Geometry check sheet. Reference: drawing and pictorial views, mm from the part's lowest x, y, z. Give positions to 0.01 mm unless a question says otherwise; leave off trailing zeros. Order: outer loops, then holes, each group sorted by start corner. A loop starts at its lowest first (then second) coordinate and runs counter-clockwise, first axis right, second up. Notation, with made-up numbers: M 85,-33.75 L 104,-33.75 A15 ccw 104,-8.75 Z; hole C -9,54 d2. An arc over 180 degrees is marked long. Answer as a JSON object with one key per item and string values. Group by question number.
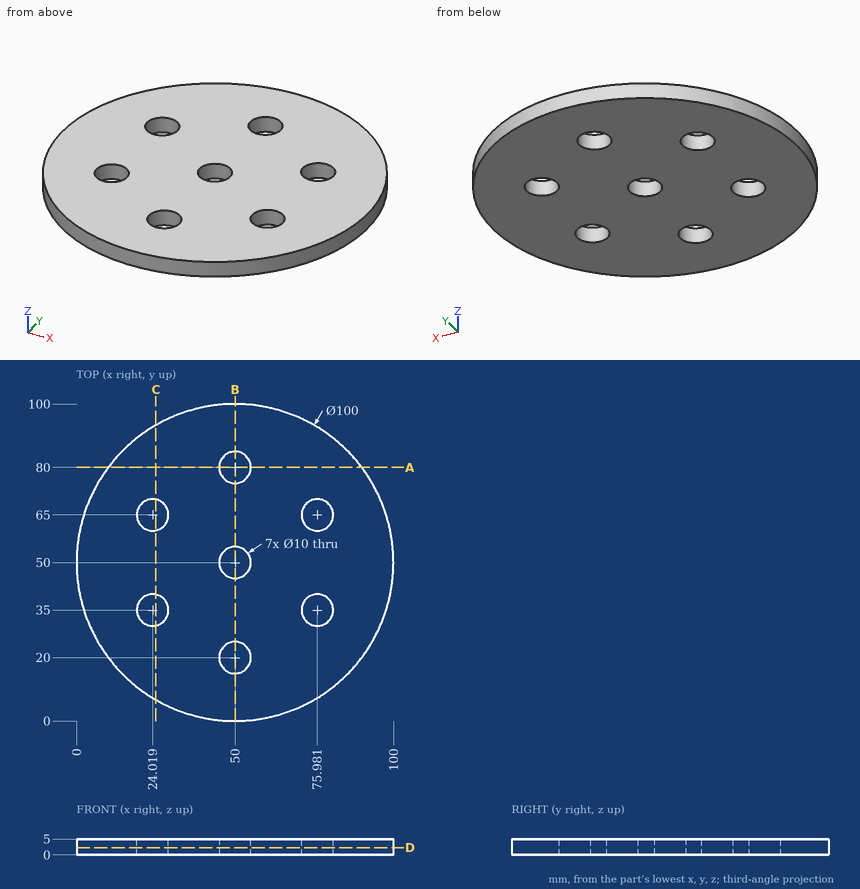
1. Cross-section at B-B (x = 50). Record the cut outline in (y, z), and give its area (3 significant figures).
2. Cross-section at C-C (x = 25). Record the cut outline in (y, z).
3. Cross-section at A-A (y = 80). Record the cut outline in (x, z), and give its area (3 significant figures).
4. Cross-section at D-D (z = 2.25). Record the cut outline in (x, y).
5. Thickness scan on line 1 along Y through (x, z) = (50, 2.1); line 2 along Y through (x, z) = (76, 2.95); line 3 along Y through (x, z) = (72.5, 1.4). Record the ranges inside material, lowest first. Write a range as [from, to].
6. Depth check by flat-ended pin: pin 1 (9 mm diameter, centred on x = 50, y = 50, fed in from -Z); pin 2 (11.5 mm diameter, centred on x = 24.02, y = 35, fed in from +Z); pin 3 (3 mm diameter, centred on y = 79, z = 2.5, fed in from -X); pin 4 (2 mm diameter, centred on x = 44, z = 3.5, fed in from +Y). Enter the tip coordinate at first touch or a pass-through.
Report:
{
 "1": {"outline": "M 0,0 L 15,0 L 15,5 L 0,5 Z; M 25,0 L 45,0 L 45,5 L 25,5 Z; M 55,0 L 75,0 L 75,5 L 55,5 Z; M 85,0 L 100,0 L 100,5 L 85,5 Z", "area": "350 mm2"},
 "2": {"outline": "M 6.7,0 L 30.1,0 L 30.1,5 L 6.7,5 Z; M 39.9,0 L 60.1,0 L 60.1,5 L 39.9,5 Z; M 69.9,0 L 93.3,0 L 93.3,5 L 69.9,5 Z"},
 "3": {"outline": "M 10,0 L 45,0 L 45,5 L 10,5 Z; M 55,0 L 90,0 L 90,5 L 55,5 Z", "area": "350 mm2"},
 "4": {"outline": "C 50,50 d100; hole C 24.02,35 d10; hole C 24.02,65 d10; hole C 50,20 d10; hole C 50,50 d10; hole C 50,80 d10; hole C 75.98,35 d10; hole C 75.98,65 d10"},
 "5": {"line 1": "y = [0, 15], [25, 45], [55, 75], [85, 100]", "line 2": "y = [7.29, 30], [40, 60], [70, 92.71]", "line 3": "y = [5.35, 31.41], [38.59, 61.41], [68.59, 94.65]"},
 "6": {"pin 1": "passes through", "pin 2": "stops at z = 5", "pin 3": "stops at x = 8.24", "pin 4": "stops at y = 99.75"}
}
